For this review, take the finished solid that the model builds, in its own axes (mm). A direction names the side the tool comes from. Coordinates: 2 decimals unless noted, no trailing zeros. Write each question's results on one line, items separated by ' | '. Start each with the question number.
```python
from build123d import *

# Parameters (mm, degrees)
SKETCH1_R                     = 7.5
BOSS_EXTRUDE1_DEPTH           = 19
BOSS_EXTRUDE1_TAPER           = 1
BOSS_EXTRUDE1_OTHER_WAY_DEPTH = 6
BOSS_EXTRUDE1_OTHER_WAY_TAPER = -1
CUT_EXTRUDE1_DEPTH            = 22.832632654
CUT_EXTRUDE1_DEPTH_BACK       = 22.832632654
CUT_EXTRUDE2_START            = -9.490788257
CUT_EXTRUDE2_OUTLINE_W        = 6.502745185
CUT_EXTRUDE2_OUTLINE_H        = 6
CUT_EXTRUDE2_DEPTH            = 9.490788257
SKETCH5_R                     = 1.5
CUT_EXTRUDE3_DEPTH            = 24.980865958
FILLET1_SIZE                  = 5
CUT_EXTRUDE4_DEPTH            = 22.796374265
CUT_EXTRUDE4_DEPTH_BACK       = 22.796374265
SKETCH6_W                     = 18.67842866
SKETCH6_H                     = 10.912736301
CUT_EXTRUDE5_DEPTH            = 19.48533084
SKETCH8_R                     = 1
CUT_EXTRUDE6_DEPTH            = 10
BOSS_EXTRUDE2_DEPTH           = 0.5


with BuildPart() as part:
    # Sketch1 → Boss-Extrude1 (new body)
    with BuildSketch(Plane(origin=(0, 0, 0), x_dir=(1, 0, 0), z_dir=(0, 1, 0))):
        Circle(SKETCH1_R)
    extrude(amount=BOSS_EXTRUDE1_DEPTH, taper=BOSS_EXTRUDE1_TAPER)

    # Sketch1 → Boss-Extrude1 other way (add)
    with BuildSketch(Plane(origin=(0, 0, 0), x_dir=(1, 0, 0), z_dir=(0, 1, 0))):
        Circle(SKETCH1_R)
    extrude(amount=-BOSS_EXTRUDE1_OTHER_WAY_DEPTH, taper=BOSS_EXTRUDE1_OTHER_WAY_TAPER)

    # Sketch3 → Cut-Extrude1 (cut, two sides: drawn at the far end of the back side and taken through both)
    with BuildSketch(Plane(origin=(0, 0, 0), x_dir=(0, 0, -1), z_dir=(1, 0, 0)).offset(-CUT_EXTRUDE1_DEPTH_BACK)):
        Polygon((-1.886057768, -6), (-1.886057768, 0), (-9.929766736, 8.043708969), (-9.929766736, -6), align=None)
    extrude(amount=CUT_EXTRUDE1_DEPTH + CUT_EXTRUDE1_DEPTH_BACK, mode=Mode.SUBTRACT)

    # Cut-Extrude2: read off the stored shape, not the designer's step
    # Cut-Extrude2 outline → Cut-Extrude2 (cut)
    with BuildSketch(Plane.XY.offset(1.886057768).offset(CUT_EXTRUDE2_START)):
        with Locations((-8.251372593, -3)):
            Rectangle(CUT_EXTRUDE2_OUTLINE_W, CUT_EXTRUDE2_OUTLINE_H)
        with Locations((8.251372593, -3)):
            Rectangle(CUT_EXTRUDE2_OUTLINE_W, CUT_EXTRUDE2_OUTLINE_H)
    extrude(amount=CUT_EXTRUDE2_DEPTH, mode=Mode.SUBTRACT)

    # Sketch5 → Cut-Extrude3 (cut, through all)
    with BuildSketch(Plane(origin=(5, 0, 0), x_dir=(0, 0, -1), z_dir=(1, 0, 0))):
        with Locations((0.613942232, -3.5)):
            Circle(SKETCH5_R)
    extrude(amount=-CUT_EXTRUDE3_DEPTH, mode=Mode.SUBTRACT)

    # Fillet1
    # a fillet whose section is not a circle: 5 mm, written as the material it takes off along each edge
    with BuildSketch(Plane(origin=(17.5, -6, 1.886057768), x_dir=(0, 0, -1), z_dir=(-1, 0, 0))) as fillet1_piece_1:
        with BuildLine():
            Bezier((FILLET1_SIZE, 0), (0, 0), (0, -FILLET1_SIZE), weights=[1, 1.5, 1])
            Line((0, -FILLET1_SIZE), (0, 0))
            Line((0, 0), (FILLET1_SIZE, 0))
        make_face()
    extrude(amount=35, mode=Mode.SUBTRACT)

    # Fillet2
    # a fillet whose section is not a circle: 10, 5 mm, written as the material it takes off along each edge
    with BuildSketch(Plane(origin=(0, 19, 0), x_dir=(1, 0, 0), z_dir=(0, 0, -1))) as fillet2_piece_1:
        with BuildLine():
            Bezier((7.341381251, 9.912737968), (7.168353766, 0), (2.342142775, 0), weights=[1, 0.818181818, 1])
            Line((2.342142775, 0), (7.168353766, 0))
            Line((7.168353766, 0), (7.341381251, 9.912737968))
        make_face()
    revolve(axis=Axis((0, 19, 0), (0, -1, 0)), mode=Mode.SUBTRACT)

    # Sketch6 → Cut-Extrude4 (cut, two sides: drawn at the far end of the back side and taken through both)
    with BuildSketch(Plane(origin=(0, 0, 0), x_dir=(0, 0, -1), z_dir=(1, 0, 0)).offset(-CUT_EXTRUDE4_DEPTH_BACK)):
        with Locations((-1.153671222, 14.54363185)):
            Rectangle(SKETCH6_W, SKETCH6_H)
    extrude(amount=CUT_EXTRUDE4_DEPTH + CUT_EXTRUDE4_DEPTH_BACK, mode=Mode.SUBTRACT)

    # Sketch7 → Cut-Extrude5 (cut, through all)
    with BuildSketch(Plane.XZ.offset(6)):
        with BuildLine():
            Line((4, -3.113942232), (4, -3.925939727))
            ThreePointArc((4, -3.925939727), (0, -5.60473039), (-4, -3.925939727))
            Line((-4, -3.925939727), (-4, -3.113942232))
            Line((-4, -3.113942232), (4, -3.113942232))
        make_face()
    extrude(amount=-CUT_EXTRUDE5_DEPTH, mode=Mode.SUBTRACT)

    # Sketch8 → Cut-Extrude6 (cut)
    with BuildSketch(Plane(origin=(0, 9.087263699, 0), x_dir=(1, 0, 0), z_dir=(0, 1, 0))):
        with Locations(Location((0, -4, 0), (0, 0, 270))):
            Circle(SKETCH8_R)
    extrude(amount=-CUT_EXTRUDE6_DEPTH, mode=Mode.SUBTRACT)

    # Sketch9 → Cut-Revolve1 (revolve, cut)
    with BuildSketch(Plane(origin=(0, 9.087263699, 0), x_dir=(1, 0, 0), z_dir=(0, 1, 0))):
        with BuildLine():
            Line((-1.5, 0), (1.5, 0))
            ThreePointArc((1.5, 0), (0, 1.5), (-1.5, 0))
        make_face()
    revolve(axis=Axis((-1.5, 9.087263699, 0), (1, 0, 0)), mode=Mode.SUBTRACT)

    # Sketch10 → Boss-Extrude2 (add)
    with BuildSketch(Plane(origin=(0, 9.087263699, 0), x_dir=(1, 0, 0), z_dir=(0, 1, 0))):
        with BuildLine():
            ThreePointArc((-1.414213562, 0.5), (-1.5, 0), (-1.414213562, -0.5))
            Line((-1.414213562, -0.5), (1.414213562, -0.5))
            ThreePointArc((1.414213562, -0.5), (1.478397839, -0.253652968), (1.5, 0))
            ThreePointArc((1.5, 0), (1.478397839, 0.253652968), (1.414213562, 0.5))
            Line((1.414213562, 0.5), (-1.414213562, 0.5))
        make_face()
    extrude(amount=-BOSS_EXTRUDE2_DEPTH)


solid = part.part
```
Q1. Insertion check: P1, Ø4, axis at x = 3, y = 7, coming from the +Z side; P2, Ø0.5, axis at x = 0, z = 0, coming from the -Y side; P3, Ø1.6, axis at x = 0, z = 4, coming from the +Y side; P4, Ø0.7, axis at x = 6.5, z = -0.5, coming from the -Y side. Each pin has a flat end and moves straight along its axis. Give the tip position at first contact, or say it passes through.
Q2. To check wall thickness, follow line 1 along Z through (x, y) = (3.5, -4.75); line 2 along Z through (x, y) = (0, 4.5); line 3 along X through (y, z) = (4, 4). State the ranges of each line that lie inside material, in increasing order.
Q3. The part is to be moulded in two halves that separate along X. For faces 4 (the face through (-6, 0, -1)), 5 (the face through (-0.969, 3.114, -7.382)), 6 (the face through (-4, 1.4, -3.5)), say which applies: pulls with the +X half, pulls with the -X half, needs draft (parallel to the pull), parting line crosses it, or undercut.
Q4. Take a section at A-A, the plane y = -3.5. Give the number of separate pieces and of enclosed holes in the cut face, then the cut area to 3 significant figures.
Q5. For faces 1 (the face through (0, 1, -3.114)), 2 (the face through (6, 0, -1)), 3 (the face through (-5, -3, -3)), list the 3-axis set-ups (+Z, -Z, +X, -X, +Y, -Y) from which the entire face can be reached by the end or side of a thin tool; tool diameter is ignored.
Results:
1) P1: z = 7.31 | P2: y = -5.67 | P3: through | P4: y = 0
2) line 1: -6.73 to -4.38, -3.11 to -1.44, 0.22 to 1.1 | line 2: -7.42 to -5.6, -3.11 to 3, 5 to 6.39 | line 3: -6.26 to -1, 1 to 6.26
3) face 4: needs draft | face 5: parting line crosses it | face 6: undercut
4) separate pieces: 2 | enclosed holes: 1 | area: 40.5 mm^2
5) face 1: +Y, -Y | face 2: +Z, -Z, +X, -Y | face 3: +Z, -Z, -X, -Y
